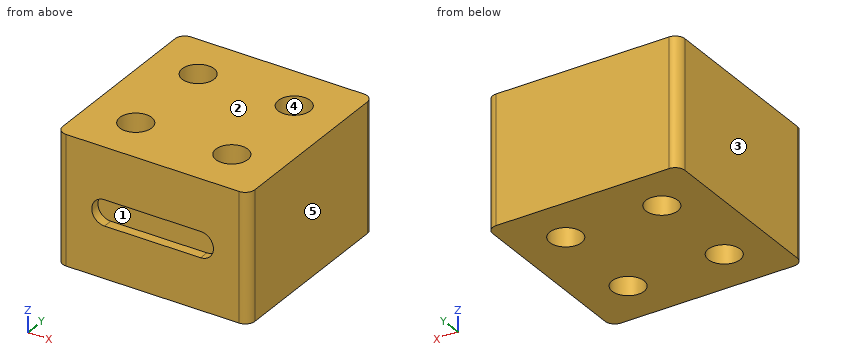
```python
from build123d import *

# Parameters (mm, degrees)
SKETCH_W     = 60
SKETCH_H     = 60
SKETCH_R     = 5
PAD_DEPTH    = 40
POCKET_DEPTH = 3
FILLET_R     = 3


with BuildPart() as part:
    # Sketch → Pad (new body)
    with BuildSketch(Plane.XY):
        Rectangle(SKETCH_W, SKETCH_H)
        with Locations((-15, 15)):
            Circle(SKETCH_R, mode=Mode.SUBTRACT)
        with Locations((15, 15)):
            Circle(SKETCH_R, mode=Mode.SUBTRACT)
        with Locations((-15, -15)):
            Circle(SKETCH_R, mode=Mode.SUBTRACT)
        with Locations((15, -15)):
            Circle(SKETCH_R, mode=Mode.SUBTRACT)
    extrude(amount=PAD_DEPTH)

    # Sketch001 (on Face4 of Pad) → Pocket (cut)
    with BuildSketch(Plane.XZ.offset(30)):
        with BuildLine():
            ThreePointArc((-15, 24), (-19, 20), (-15, 16))
            Line((-15, 16), (15, 16))
            ThreePointArc((15, 16), (19, 20), (15, 24))
            Line((-15, 24), (15, 24))
        make_face()
    extrude(amount=-POCKET_DEPTH, mode=Mode.SUBTRACT)

    # Fillet
    fillet_edges = [part.edges().sort_by_distance(p)[0] for p in [
        (30, -30, 20),
        (30, 30, 20),
        (-30, -30, 20),
        (-30, 30, 20),
    ]]
    fillet(fillet_edges, radius=FILLET_R)


solid = part.part
```
CAD build for the part. Positions are in the model's coordinates, mm. Face numbers are marked on the shaded views. A direction names the side the tool comes from. Round coordinates to 2 decimals unless told otherwise and drop trailing zeros. Write each loop counter-clockwise with the first axis right and the second up, starting at its lowest first coordinate (ties: lowest second). Pieces come first, ordered by that corner, then holes. Notation, with made-up numbers: (31, 84.5) - (64, 84.5) arc R16 cw to (64, 99.5) - close; hole circle Ø7 at (3.5, 59). An arc over 180 degrees is marked (long way). Return JSON: item names as keys, results as strings. Group by question number.
Item 1: 3-axis set-ups, long thin cutter, end or side, ignore diameter. For the marked faces 1 and 2: which of +Z, -Z, +X, -X, +Y, -Y reach the whole face in a straight line?
Item 2: Mould opens along X. For the marked faces 3, 4 and 5 say: +X half, -X half, draft (parallel to the pull), parting line (faces both ways), or undercut.
Item 3: Band-saw the part on D-D on z = 20. List the corners of the cut face in (x, y).
Item 4: Band-saw the part on A-A on y = 15. List the corners of the cut face in (x, z), plus the area to 3 significant figures.
Item 5: Band-saw the part on C-C on x = 12.5. List the corners of the cut face in (y, z).
Item 6: Flat gauge pin, fed straight in: pin 1 Ø2 at (x, z) = (-7.5, 20.5) entering from -Y. Where does the tip first touch, or does it go through?
Item 7: Probe probe 1 along Y at (x, z) = (15, 16.5); probe 2 along Z at (x, y) = (0.5, -27.5); probe 3 along Y at (x, z) = (-15, 11). List the from-to ranges inside material, lowest first.
Item 8: Band-saw the part on B-B on z = 26. List the corners of the cut face in (x, y).
Resolved:
{
 "1": {"face 1": "-Y", "face 2": "+Z, +X, -X, +Y, -Y"},
 "2": {"face 3": "-X half", "face 4": "undercut", "face 5": "+X half"},
 "3": {"outline": "(-30, -27) arc R3 ccw to (-27, -30) - (-19, -30) - (-19, -27) - (19, -27) - (19, -30) - (27, -30) arc R3 ccw to (30, -27) - (30, 27) arc R3 ccw to (27, 30) - (-27, 30) arc R3 ccw to (-30, 27) - close; hole circle Ø10 at (-15, -15); hole circle Ø10 at (-15, 15); hole circle Ø10 at (15, -15); hole circle Ø10 at (15, 15)"},
 "4": {"outline": "(-30, 0) - (-20, 0) - (-20, 40) - (-30, 40) - close; (-10, 0) - (10, 0) - (10, 40) - (-10, 40) - close; (20, 0) - (30, 0) - (30, 40) - (20, 40) - close", "area": "1,600 mm²"},
 "5": {"outline": "(-30, 0) - (-19.33, 0) - (-19.33, 40) - (-30, 40) - (-30, 24) - (-27, 24) - (-27, 16) - (-30, 16) - close; (-10.67, 0) - (10.67, 0) - (10.67, 40) - (-10.67, 40) - close; (19.33, 0) - (30, 0) - (30, 40) - (19.33, 40) - close"},
 "6": {"pin 1": "stops at y = -27"},
 "7": {"probe 1": "y = -27 to -20, -10 to 10, 20 to 30", "probe 2": "z = 0 to 16, 24 to 40", "probe 3": "y = -30 to -20, -10 to 10, 20 to 30"},
 "8": {"outline": "(-30, -27) arc R3 ccw to (-27, -30) - (27, -30) arc R3 ccw to (30, -27) - (30, 27) arc R3 ccw to (27, 30) - (-27, 30) arc R3 ccw to (-30, 27) - close; hole circle Ø10 at (-15, -15); hole circle Ø10 at (-15, 15); hole circle Ø10 at (15, -15); hole circle Ø10 at (15, 15)"}
}
